Source: CAD feature listing. Evaluate the final solid. Frame: model axes, mm. A direction names the side the tool comes from. Give positions to 0.01 mm unless a question says otherwise; leave off trailing zeros. Order: outer loops, then holes, each group sorted by start corner. A loop starts at its lowest first (then second) coordinate and runs counter-clockwise, first axis right, second up. Notation, with made-up numbers: (85, -18) - (93, -18) arc R30 cw to (93, 13) - close; hole circle Ø9 at (14, 60.5). An arc over 180 degrees is marked (long way). Answer as CSV lines item,"result".
```python
from build123d import *

# Parameters (mm, degrees)
SKETCH_1_R          = 12.2
EXTRUDE_1_DEPTH     = 30.8
FILLET_1_R          = 2
SKETCH_2_R          = 3.25
EXTRUDE_2_DEPTH     = 1.7
SKETCH_5_R          = 1
EXTRUDE_4_DEPTH     = 4
SKETCH_7_W          = 1.851248616
SKETCH_7_H          = 0.354328631
CUT_EXTRUDE_1_DEPTH = 1
SKETCH_8_W          = 0.317488429
SKETCH_8_H          = 1.793967755
CUT_EXTRUDE_2_DEPTH = 1
SKETCH_10_W         = 0.364887613
SKETCH_10_H         = 1.860802793
CUT_EXTRUDE_4_DEPTH = 1
SKETCH_11_W         = 1.9755237
SKETCH_11_H         = 0.380671715
CUT_EXTRUDE_5_DEPTH = 1


with BuildPart() as part:
    # 草图1 → 凸台-拉伸1 (new body)
    with BuildSketch(Plane.XY):
        with Locations(Location((0, 0, 0), (0, 0, 180))):
            Circle(SKETCH_1_R)
    extrude(amount=EXTRUDE_1_DEPTH)

    # 圆角1
    fillet_1_edges = [part.edges().sort_by_distance(p)[0] for p in [
        (12.2, 0, 30.8),
    ]]
    fillet(fillet_1_edges, radius=FILLET_1_R)

    # 草图2 → 凸台-拉伸2 (add)
    with BuildSketch(Plane(origin=(0, 0, 0), x_dir=(-1, 0, 0), z_dir=(0, 0, -1))):
        Circle(SKETCH_2_R)
    extrude(amount=EXTRUDE_2_DEPTH)

    # 草图5 → 凸台-拉伸4 (add)
    with BuildSketch(Plane(origin=(0, 0, 0), x_dir=(-1, 0, 0), z_dir=(0, 0, -1))):
        with Locations(Location((0, -8.5, 0), (0, 0, 180))):
            Circle(SKETCH_5_R)
        with Locations(Location((0, 8.5, 0), (0, 0, 180))):
            Circle(SKETCH_5_R)
    extrude(amount=EXTRUDE_4_DEPTH)

    # 草图7 → 切除-拉伸1 (cut)
    with BuildSketch(Plane(origin=(0, 0, 0), x_dir=(-1, 0, 0), z_dir=(0, 0, -1))):
        with Locations((-8.515796524, 0.01329556)):
            Rectangle(SKETCH_7_W, SKETCH_7_H)
    extrude(amount=-CUT_EXTRUDE_1_DEPTH, mode=Mode.SUBTRACT)

    # 草图8 → 切除-拉伸2 (cut)
    with BuildSketch(Plane(origin=(0, 0, 0), x_dir=(-1, 0, 0), z_dir=(0, 0, -1))):
        with Locations((-8.493083651, -0.013515685)):
            Rectangle(SKETCH_8_W, SKETCH_8_H)
    extrude(amount=-CUT_EXTRUDE_2_DEPTH, mode=Mode.SUBTRACT)

    # 草图10 → 切除-拉伸4 (cut)
    with BuildSketch(Plane(origin=(0, 0, 0), x_dir=(-1, 0, 0), z_dir=(0, 0, -1))):
        with Locations((8.376136345, -0.021771447)):
            Rectangle(SKETCH_10_W, SKETCH_10_H)
    extrude(amount=-CUT_EXTRUDE_4_DEPTH, mode=Mode.SUBTRACT)

    # 草图11 → 切除-拉伸5 (cut)
    with BuildSketch(Plane(origin=(0, 0, 0), x_dir=(-1, 0, 0), z_dir=(0, 0, -1))):
        with Locations((8.368475893, -0.042969493)):
            Rectangle(SKETCH_11_W, SKETCH_11_H)
    extrude(amount=-CUT_EXTRUDE_5_DEPTH, mode=Mode.SUBTRACT)


solid = part.part
```
(1) Contact query for flat-ended pins moving along their axis: pin 1 (3 mm diameter, centred on y = 4.5, z = 26.5, fed in from +X); pin 2 (1 mm diameter, centred on y = -0.5, z = 16, fed in from +X); pin 3 (0.6 mm diameter, centred on x = -9, z = 0.5, fed in from -Y); pin 4 (4 mm diameter, centred on y = -9.5, z = 10.5, fed in from -X). Output: stop coordinate, or through.
Completed:
pin 1,"x = 11.83"
pin 2,"x = 12.2"
pin 3,"y = -8.55"
pin 4,"x = -9.62"
(2) Mould query, pull axis Y, two halves, no side actions, for faces 1 (the flat face through (-7.8, 0.147, 0.5)), 2 (the flat face through (0, 0, 30.8)), 3 (the cylindrical face through (12.19, -0.54, 14.2)). Classes: released by +Y, released by -Y, zero draft, split by the parting line, or undercut.
Completed:
face 1,"undercut"
face 2,"zero draft"
face 3,"split by the parting line"
(3) Cut plane A-A (x = 0). Return loops of the section in (y, z), then the cut area to 3 significant figures.
Completed:
outline,"(-12.2, 0) - (-9.5, 0) - (-9.5, -4) - (-7.5, -4) - (-7.5, 0) - (-3.25, 0) - (-3.25, -1.7) - (3.25, -1.7) - (3.25, 0) - (7.5, 0) - (7.5, -4) - (9.5, -4) - (9.5, 0) - (12.2, 0) - (12.2, 28.8) arc R2 ccw to (10.2, 30.8) - (-10.2, 30.8) arc R2 ccw to (-12.2, 28.8) - close"
area,"777 mm²"
(4) Cut plane B-B (z = 11). Return loops of the section in (x, y).
Completed:
outline,"circle Ø24.4 at (0, 0)"
(5) Ray query, line 1 (Z direction, x = 3.75, y = -3.5); line 2 (Z direction, x = 1, y = -2.25); line 3 (Y direction, x = -2.5, z = 10). Return the intervals inside material, ascending. Write a range as from..to.
Completed:
line 1,"0..30.8"
line 2,"-1.7..30.8"
line 3,"-11.94..11.94"
(6) Access query for faces 4 (the flat face through (0, 0, -1.7)), 5 (the flat face through (0, 8, -4)), 6 (the flat face through (-3, 3, 0)). Directions: +Z, -Z, +X, -X, +Y, -Y. A direction counts if a zero-diameter tool reaches every point of the face in a straight line with its end or side. Return the directions, or none.
Completed:
face 4,"-Z, +X, -X"
face 5,"-Z, +X, -X, +Y, -Y"
face 6,"-Z"
